The listing builds one solid part. Answer for the finished solid, in the listing's coordinates (mm). Face numbers are marked on the shaded views. Give positions to 0.01 mm unless a question says otherwise; leave off trailing zeros. Write each loop counter-clockwise with the first axis right and the second up, starting at its lowest first coordinate (ties: lowest second). Pieces come first, ordered by that corner, then holes. Notation, with made-up numbers: (1.5, 73.5) - (9.5, 73.5) arc R31 ccw to (9.5, 100.5) - close; hole circle Ø8 at (80, 21). An arc over 180 degrees is marked (long way). Return JSON: item names as keys, results as strings.
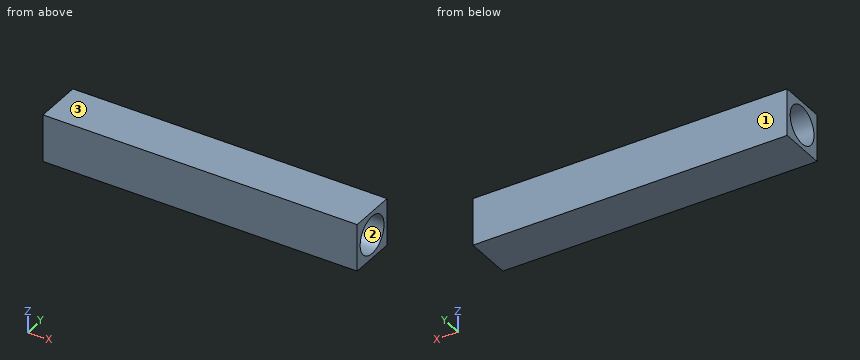
from build123d import *

# Parameters (mm, degrees)
SKETCH1_W           = 95.25
SKETCH1_H           = 95.25
SKETCH1_R           = 38.1
BOSS_EXTRUDE1_DEPTH = 317.5


with BuildPart() as part:
    # Sketch1 → Boss-Extrude1 (new, symmetric)
    with BuildSketch(Plane(origin=(0, 0, 0), x_dir=(0, 0, -1), z_dir=(1, 0, 0))):
        with Locations((-47.625, 47.625)):
            Rectangle(SKETCH1_W, SKETCH1_H)
        with Locations(Location((-47.625, 47.625, 0), (0, 0, 180))):
            Circle(SKETCH1_R, mode=Mode.SUBTRACT)
    extrude(amount=BOSS_EXTRUDE1_DEPTH, both=True)


solid = part.part
Item 1: A cutting plane is placed at C-C on x = -33. Determine the outline of the cut face in (y, z) (3 decimals), then the cut area to 3 significant figures.
Answer below:
{"outline": "(0, 0) - (95.25, 0) - (95.25, 95.25) - (0, 95.25) - close; hole circle Ø76.2 at (47.625, 47.625)", "area": "4,510 mm²"}
Item 2: Consider L1, parallel to Z at x = -76, y = 49; L2, parallel to Y at x = -17, z = 48; L3, parallel to Z at x = 92, y = 55. Determine where each line is inside the solid, lowest interval first.
Answer below:
{"L1": "z = 0 to 9.55, 85.7 to 95.25", "L2": "y = 0 to 9.53, 85.72 to 95.25", "L3": "z = 0 to 10.25, 85 to 95.25"}
Item 3: A cutting plane is placed at B-B on z = 67.5. Determine the outline of the cut face in (x, y), then the cut area to 3 significant figures.
Answer below:
{"outline": "(-317.5, 0) - (317.5, 0) - (317.5, 15.12) - (-317.5, 15.12) - close; (-317.5, 80.13) - (317.5, 80.13) - (317.5, 95.25) - (-317.5, 95.25) - close", "area": "19,200 mm²"}
Item 4: A flat-ended cylindrical pin translates along its axis: P1, Ø2, axis at x = 104, z = 72, coming from the -Y side. Find the tip coordinate at first contact, or state that the pin passes through.
Answer below:
{"P1": "stops at y = 0"}
Item 5: The mould has two halves that part along Y. Classify the marked faces 1, 2 and 3: +Y half, -Y half, draft (parallel to the pull), parting line (faces both ways), or undercut.
Answer below:
{"face 1": "+Y half", "face 2": "undercut", "face 3": "draft"}
Item 6: A cutting plane is placed at A-A on y = 58. Determine the outline of the cut face in (x, z).
Answer below:
{"outline": "(-317.5, 0) - (317.5, 0) - (317.5, 10.96) - (-317.5, 10.96) - close; (-317.5, 84.29) - (317.5, 84.29) - (317.5, 95.25) - (-317.5, 95.25) - close"}
